```python
from build123d import *

# Parameters (mm, degrees)
EXTRUDE_1_DEPTH     = 38
EXTRUDE_2_DEPTH     = 1.5
SKETCH_3_W          = 34
SKETCH_3_H          = 9.5
CUT_EXTRUDE_1_DEPTH = 51.831215803
SKETCH_6_R          = 2
CUT_EXTRUDE_2_DEPTH = 1.5
CUT_EXTRUDE_3_REACH = 51.346
SKETCH_7_R          = 1.5


with BuildPart() as part:
    # 草图1 → 凸台-拉伸1 (new body)
    with BuildSketch(Plane(origin=(0, 0, 0), x_dir=(0, 0, -1), z_dir=(1, 0, 0))):
        with BuildLine():
            Line((-3.998463992, 0.110840888), (-4.75, -27))
            Line((-4.75, -27), (4.75, -27))
            Line((4.75, -27), (3.998463992, 0.110840888))
            ThreePointArc((3.998463992, 0.110840888), (0, 4), (-3.998463992, 0.110840888))
        make_face()
    extrude(amount=EXTRUDE_1_DEPTH)

    # 草图4 → 凸台-拉伸2 (add)
    with BuildSketch(Plane.XZ.offset(27)):
        with BuildLine():
            Line((6.5, 4.75), (0, 4.75))
            Line((0, 4.75), (0, -4.75))
            Line((0, -4.75), (6.5, -4.75))
            ThreePointArc((6.5, -4.75), (19, -13.37207912), (31.5, -4.75))
            Line((31.5, -4.75), (38, -4.75))
            Line((38, -4.75), (38, 4.75))
            Line((38, 4.75), (31.5, 4.75))
            ThreePointArc((31.5, 4.75), (19, 13.37207912), (6.5, 4.75))
        make_face()
    extrude(amount=EXTRUDE_2_DEPTH)

    # 草图3 → 切除-拉伸1 (cut, through all)
    with BuildSketch(Plane.XZ.offset(27)):
        with Locations((19, 0)):
            Rectangle(SKETCH_3_W, SKETCH_3_H)
    extrude(amount=-CUT_EXTRUDE_1_DEPTH, mode=Mode.SUBTRACT)

    # 草图6 → 切除-拉伸2 (cut)
    with BuildSketch(Plane.XZ.offset(28.5)):
        with Locations(Location((19, 0, 0), (0, 0, 270))):
            Circle(SKETCH_6_R)
        with BuildLine():
            Line((6, 1.5), (11, 1.5))
            ThreePointArc((11, 1.5), (12.5, 0), (11, -1.5))
            Line((11, -1.5), (6, -1.5))
            ThreePointArc((6, -1.5), (4.5, 0), (6, 1.5))
        make_face()
        with BuildLine():
            Line((32, 1.5), (27, 1.5))
            ThreePointArc((27, 1.5), (25.5, 0), (27, -1.5))
            Line((27, -1.5), (32, -1.5))
            ThreePointArc((32, -1.5), (33.5, 0), (32, 1.5))
        make_face()
        with BuildLine():
            ThreePointArc((24, 8.660254038), (19, 10), (14, 8.660254038))
            ThreePointArc((14, 8.660254038), (13.633974596, 7.294228634), (15, 6.92820323))
            ThreePointArc((15, 6.92820323), (19, 8), (23, 6.92820323))
            ThreePointArc((23, 6.92820323), (24.366025404, 7.294228634), (24, 8.660254038))
        make_face()
        with BuildLine():
            ThreePointArc((24, -8.660254038), (24.366025404, -7.294228634), (23, -6.92820323))
            ThreePointArc((23, -6.92820323), (19, -8), (15, -6.92820323))
            ThreePointArc((15, -6.92820323), (13.633974596, -7.294228634), (14, -8.660254038))
            ThreePointArc((14, -8.660254038), (19, -10), (24, -8.660254038))
        make_face()
    extrude(amount=-CUT_EXTRUDE_2_DEPTH, mode=Mode.SUBTRACT)

    # 切除-拉伸3: up to this face of the body (flat: up to its plane)
    cut_extrude_3_end = Plane(part.part.faces().sort_by_distance((38, -13.180930024, 0))[0])
    # 草图7 → 切除-拉伸3 (cut, up to the picked face)
    with BuildSketch(Plane.ZY, mode=Mode.PRIVATE) as cut_extrude_3_sk1:
        with Locations(Location((0, 0, 0), (0, 0, 180))):
            Circle(SKETCH_7_R)
    cut_extrude_3_tool1 = split(extrude(cut_extrude_3_sk1.sketch, amount=-CUT_EXTRUDE_3_REACH, mode=Mode.PRIVATE), bisect_by=cut_extrude_3_end, keep=Keep.BOTH, mode=Mode.PRIVATE)
    add(cut_extrude_3_tool1.solids().sort_by(Axis((0, 0, 0), (1, 0, 0)))[0], mode=Mode.SUBTRACT)


solid = part.part
```
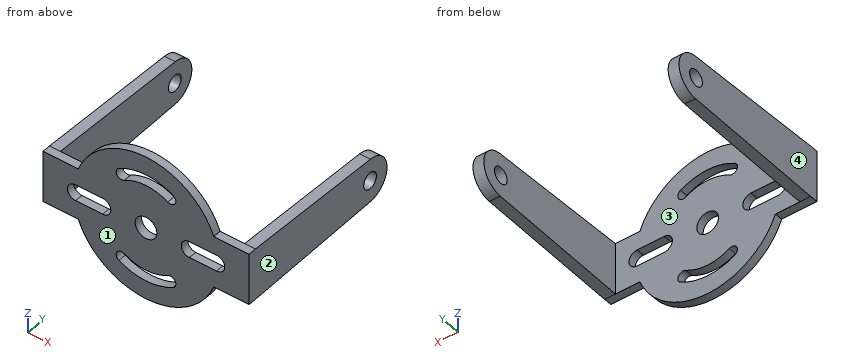
Input: part model. Units: mm. Frame: model coordinates. Face numbers are marked on the shaded views. Round coordinates to 2 decimals unless told otherwise and drop trailing zeros. Loops run counter-clockwise (first coordinate to the right, second up) from the corner with the lowest first, then second, coordinate; pieces in that order, holes last. Notation, with made-up numbers: (-33.75, -16.75) -> (-3.75, -16.75) arc R18 ccw to (-3.75, -7.75) -> close; hole circle Ø6 at (6, 66.25). An arc over 180 degrees is marked (long way). Write each question's results on one line, items separated by ' | '.
1. Ray query, line 1 (X direction, y = -27.65, z = 0); line 2 (Y direction, x = 36.6, z = 0); line 3 (X direction, y = -22, z = -1.25). Return the intervals inside material, ascending. Write a range as from..to.
Geometry results:
line 1: 0..4.5, 12.5..17, 21..25.5, 33.5..38 | line 2: -28.5..-1.5, 1.5..4 | line 3: 0..2, 36..38
2. Section D-D (x = 23.5). Return loops of the section in (y, z), and give its area (3 significant figures).
Geometry results:
outline: (-28.5, -12.59) -> (-27, -12.59) -> (-27, -8.93) -> (-28.5, -8.93) -> close; (-28.5, -6.79) -> (-27, -6.79) -> (-27, 6.79) -> (-28.5, 6.79) -> close; (-28.5, 8.93) -> (-27, 8.93) -> (-27, 12.59) -> (-28.5, 12.59) -> close | area: 31.4 mm2
3. Mould query, pull axis X, two halves, no side actions, for the marked faces 1, 2, 3 and 4. Classes: +X half, -X half, draft (parallel to the pull), parting line (faces both ways), or undercut.
Geometry results:
face 1: draft | face 2: +X half | face 3: undercut | face 4: -X half
4. Section A-A (z = 0). Return loops of the section in (x, y).
Geometry results:
outline: (0, -28.5) -> (4.5, -28.5) -> (4.5, -27) -> (2, -27) -> (2, -1.5) -> (0, -1.5) -> close; (0, 1.5) -> (2, 1.5) -> (2, 4) -> (0, 4) -> close; (12.5, -28.5) -> (17, -28.5) -> (17, -27) -> (12.5, -27) -> close; (21, -28.5) -> (25.5, -28.5) -> (25.5, -27) -> (21, -27) -> close; (33.5, -28.5) -> (38, -28.5) -> (38, -1.5) -> (36, -1.5) -> (36, -27) -> (33.5, -27) -> close; (36, 1.5) -> (38, 1.5) -> (38, 4) -> (36, 4) -> close
5. First-contact query: P1, Ø10, axis at x = 9, z = -7.5, coming from the +Y side; P2, Ø0.8, axis at x = 34.5, y = -27.5, coming from the +Z side; P3, Ø1.2, axis at x = 30, y = -28, coming from the +Z side; P4, Ø3.5, axis at y = 0, z = 0, coming from the +X side. Flat tips, straight axial feed; report the tip coordinate or a pass-through.
Geometry results:
P1: y = -27 | P2: z = 4.75 | P3: z = 8.41 | P4: x = 38
6. Section C-C (y = -2). Return loops of the section in (x, z), and give its area (3 significant figures).
Geometry results:
outline: (0, -4.06) -> (2, -4.06) -> (2, 4.06) -> (0, 4.06) -> close; (36, -4.06) -> (38, -4.06) -> (38, 4.06) -> (36, 4.06) -> close | area: 32.5 mm2
7. Section B-B (x = 19). Return loops of the section in (y, z), and give its area (3 significant figures).
Geometry results:
outline: (-28.5, -13.37) -> (-27, -13.37) -> (-27, -10) -> (-28.5, -10) -> close; (-28.5, -8) -> (-27, -8) -> (-27, -2) -> (-28.5, -2) -> close; (-28.5, 2) -> (-27, 2) -> (-27, 8) -> (-28.5, 8) -> close; (-28.5, 10) -> (-27, 10) -> (-27, 13.37) -> (-28.5, 13.37) -> close | area: 28.1 mm2
